Part model, mm, in its own coordinate system. A direction names the side the tool comes from. Round coordinates to 2 decimals unless told otherwise and drop trailing zeros. Loops run counter-clockwise (first coordinate to the right, second up) from the corner with the lowest first, then second, coordinate; pieces in that order, holes last. Notation, with made-up numbers: (-3, 87.25) - (27, 87.25) arc R8 ccw to (27, 92.25) - close; hole circle Ø3 at (61, -18). An arc over 180 degrees is marked (long way). Write each question's results on one line, items separated by ' | '. Start each with the question number.
(1) Cut at A-A, the plane z = -9. List the corners of the cut face in (x, y).
(2) Cut at C-C, the plane z = 11.5. List the corners of the cut face in (x, y).
(3) Flat gauge pins, fed straight in: P1, Ø10, axis at x = 10, y = -15, coming from the +Z side; P2, Ø6, axis at x = -57, y = -17, coming from the -Z side; P3, Ø15, axis at x = 9.5, z = 5.5, coming from the +Y side. Where does each tip first touch, or does it go through?
(4) Mould opens along Y. For faces 5 (the face through (-19.3, 10, 8)), 6 (the face through (7, 25.45, -6)), 7 (the face through (-46, 9.9, -7)) say: released by +Y, released by -Y, zero draft, split by the parting line, or undercut.
(5) Tool access for faces 1 (the face through (7, 27.99, -6)), 2 (the face through (38.243, 27, -6)), 3 (the face through (-17.829, -19, -6)), 4 (the face through (46, -16.053, -6)): list every direction of +Z, -Z, +X, -X, +Y, -Y with a clear straight run to the whole face (end or side of a thin tool).
(6) Cut at B-B, the plane x = -27. List the corners of the cut face in (y, z).
(7) Drill centre lines: L1, parallel to X at y = -20.15, z = -11.95; L2, parallel to Z at x = -2, y = -8.5; L3, parallel to Z at x = -27.5, y = -3. Where is each one in solid material? Low to high.
(8) Cut at D-D, the plane x = -1.5. List the corners of the cut face in (y, z), then the cut area to 3 significant figures.
from build123d import *

# Parameters (mm, degrees)
ESBO_O1_W                 = 100
ESBO_O1_H                 = 60
ESBO_O1_R                 = 1.85
RESSALTO_EXTRUS_O1_DEPTH  = 1.7
ESBO_O2_W                 = 60
ESBO_O2_H                 = 15
ESBO_O2_W_2               = 40
RESSALTO_EXTRUS_O2_DEPTH  = 13.6
RESSALTO_EXTRUS_O6_START  = 11.6
ESBO_O3_W                 = 100
ESBO_O3_H                 = 53
ESBO_O3_R                 = 1.85
RESSALTO_EXTRUS_O6_DEPTH  = 1.5
ESBO_O4_W                 = 62.184169383
ESBO_O4_H                 = 2.54
ESBO_O4_W_2               = 5.08
ESBO_O4_H_2               = 42.957805244
ESBO_O4_W_3               = 56.07185462
RESSALTO_EXTRUS_O8_DEPTH  = 11.6
ESBO_O6_W                 = 21
ESBO_O6_H                 = 20
RESSALTO_EXTRUS_O9_DEPTH  = 16
ESBO_O7_W                 = 23.246964405
ESBO_O7_H                 = 12
RESSALTO_EXTRUS_O10_DEPTH = 10


with BuildPart() as part:
    # Esbo_o1 → Ressalto-extrus_o1 (new body)
    with BuildSketch(Plane.XY):
        Rectangle(ESBO_O1_W, ESBO_O1_H)
        with Locations((-34.15, 27.15)):
            Circle(ESBO_O1_R, mode=Mode.SUBTRACT)
        with Locations((-35.55, -20.15)):
            Circle(ESBO_O1_R, mode=Mode.SUBTRACT)
        with Locations((44.65, -19.95)):
            Circle(ESBO_O1_R, mode=Mode.SUBTRACT)
    extrude(amount=RESSALTO_EXTRUS_O1_DEPTH)

    # Esbo_o2 → Ressalto-extrus_o2 (add)
    with BuildSketch(Plane.XY.offset(1.7)):
        with Locations((10.7, -12.2)):
            Rectangle(ESBO_O2_W, ESBO_O2_H)
        with Locations((0.7, 10.2)):
            Rectangle(ESBO_O2_W_2, ESBO_O2_H)
    extrude(amount=RESSALTO_EXTRUS_O2_DEPTH)



with BuildPart() as body_2:
    # Esbo_o3 → Ressalto-extrus_o6 (new body)
    with BuildSketch(Plane(origin=(0, 0, 0), x_dir=(-1, 0, 0), z_dir=(0, 0, -1)).offset(RESSALTO_EXTRUS_O6_START)):
        with Locations((0, 4.4)):
            Rectangle(ESBO_O3_W, ESBO_O3_H)
        with Locations(Location((-44.65, -19.95, 0), (0, 0, 180))):
            Circle(ESBO_O3_R, mode=Mode.SUBTRACT)
        with Locations(Location((34.15, 27.15, 0), (0, 0, 180))):
            Circle(ESBO_O3_R, mode=Mode.SUBTRACT)
        with Locations(Location((35.55, -20.15, 0), (0, 0, 180))):
            Circle(ESBO_O3_R, mode=Mode.SUBTRACT)
    extrude(amount=RESSALTO_EXTRUS_O6_DEPTH)


with BuildPart() as part_1:
    add(part.part)

    add(body_2.part)  # Ressalto-extrus_o8 merges body 2
    # Esbo_o4 → Ressalto-extrus_o8 (add)
    with BuildSketch(Plane.XY.offset(-11.6)):
        with Locations((7.150543675, 26.719832293)):
            Rectangle(ESBO_O4_W, ESBO_O4_H)
        with Locations((45.784919315, 5.42627648)):
            Rectangle(ESBO_O4_W_2, ESBO_O4_H_2)
        with Locations((10.206701056, -18.689881399)):
            Rectangle(ESBO_O4_W_3, ESBO_O4_H)
    extrude(amount=RESSALTO_EXTRUS_O8_DEPTH)

    # Esbo_o6 → Ressalto-extrus_o9 (add)
    with BuildSketch(Plane.XY.offset(1.7)):
        with Locations((-51.5, -19)):
            Rectangle(ESBO_O6_W, ESBO_O6_H)
    extrude(amount=RESSALTO_EXTRUS_O9_DEPTH)

    # Esbo_o7 → Ressalto-extrus_o10 (add)
    with BuildSketch(Plane.XY.offset(-11.6)):
        with Locations((-45.376517798, 15.9)):
            Rectangle(ESBO_O7_W, ESBO_O7_H)
    extrude(amount=RESSALTO_EXTRUS_O10_DEPTH)


solid = part_1.part
A:
1) outline: (-57, 9.9) - (-33.75, 9.9) - (-33.75, 21.9) - (-57, 21.9) - close; (-23.94, 25.45) - (38.24, 25.45) - (38.24, 27.99) - (-23.94, 27.99) - close; (-17.83, -19.96) - (38.24, -19.96) - (38.24, -17.42) - (-17.83, -17.42) - close; (43.24, -16.05) - (48.32, -16.05) - (48.32, 26.91) - (43.24, 26.91) - close
2) outline: (-62, -29) - (-41, -29) - (-41, -9) - (-62, -9) - close; (-19.3, -19.7) - (40.7, -19.7) - (40.7, -4.7) - (-19.3, -4.7) - close; (-19.3, 2.7) - (20.7, 2.7) - (20.7, 17.7) - (-19.3, 17.7) - close
3) P1: z = 15.3 | P2: z = 1.7 | P3: y = 30
4) face 5: zero draft | face 6: undercut | face 7: released by -Y
5) face 1: +X, -X, +Y | face 2: +Y, -Y | face 3: -X, -Y | face 4: +X, -X, -Y
6) outline: (-30, 0) - (30, 0) - (30, 1.7) - (-30, 1.7) - close; (-22.1, -13.1) - (30.9, -13.1) - (30.9, -11.6) - (-22.1, -11.6) - close
7) L1: -50 to -37.4, -33.7 to 42.81, 46.49 to 50 | L2: -13.1 to -11.6, 0 to 15.3 | L3: -13.1 to -11.6, 0 to 1.7
8) outline: (-30, 0) - (-19.96, 0) - (-19.96, -11.6) - (-22.1, -11.6) - (-22.1, -13.1) - (30.9, -13.1) - (30.9, -11.6) - (27.99, -11.6) - (27.99, 0) - (30, 0) - (30, 1.7) - (17.7, 1.7) - (17.7, 15.3) - (2.7, 15.3) - (2.7, 1.7) - (-4.7, 1.7) - (-4.7, 15.3) - (-19.7, 15.3) - (-19.7, 1.7) - (-30, 1.7) - close; hole (-17.42, -11.6) - (25.45, -11.6) - (25.45, 0) - (-17.42, 0) - close | area: 648 mm2
